The listing builds one solid part. Answer for the finished solid, in the listing's coordinates (mm). Face numbers are marked on the shaded views. A direction names the side the tool comes from. Round coordinates to 2 decimals unless told otherwise and drop trailing zeros. Write each loop counter-clockwise with the first axis right and the second up, starting at its lowest first coordinate (ties: lowest second). Pieces come first, ordered by that corner, then holes.
(1) Each of these flat-tipped pins is pushed along its axis until it touches: pin 1 Ø1 at (x, z) = (-41.5, -9.5) entering from +Y; pin 2 Ø8 at (y, z) = (-8.5, 13) entering from +X. Where does it stop, or does it pass through?
(2) For the marked faces 1 and 2, determine the directions among +Z, -Z, +X, -X, +Y, -Y from which every point of the face is accessible in a straight line to the end or side of a thin tool.
(3) A cutting plane is placed at D-D, the plane x = -24. Give the vertices of the cut face in (y, z).
(4) Find the intervals of material crossed by probe 1 along Z at (x, y) = (30.5, -5.25); probe 2 along Y at (x, z) = (38, 11); probe 3 along Y at (x, z) = (0, -23), in increasing order.
(5) A cutting plane is placed at A-A, the plane z = -8.5. Give the vertices of the cut face in (x, y), and give its area (3 significant figures).
(6) A cutting plane is placed at B-B, the plane y = -5.5. Give the vertices of the cut face in (x, z), and give its area (3 significant figures).
(7) The mould has two halves that part along Y. Classify the marked faces 3, 4 and 5: +Y half, -Y half, draft (parallel to the pull), parting line (faces both ways), or undercut.
(8) A cutting plane is placed at C-C, the plane x = 38.5. Give the vertices of the cut face in (y, z).
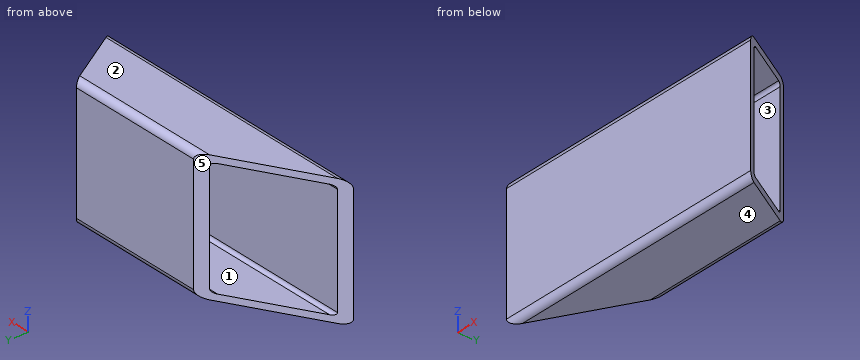
from build123d import *

# Parameters (mm, degrees)
F0_W     = 112.7125
F0_H     = 50.8
F1_DEPTH = 12.7
F2_T     = -2.54
F4_DEPTH = 50.801
F6_DEPTH = 50.801
F7_R     = 2.54
F8_R     = 1.27


with BuildPart() as f1:
    # F0 (on Front) → F1 (new body, symmetric)
    with BuildSketch(Plane.XZ):
        Rectangle(F0_W, F0_H)
    extrude(amount=F1_DEPTH, both=True)

    # F2
    f2_openings = [f1.faces().sort_by_distance(p)[0] for p in [
        (-56.35625, 0, 0),
        (56.35625, 0, 0),
    ]]
    offset(amount=F2_T, openings=f2_openings)

    # F3 (on face) → F4 (cut, through all)
    with BuildSketch(Plane(origin=(0, 0, -25.4), x_dir=(1, 0, 0), z_dir=(0, 0, -1))):
        Polygon((-12.3621594878, -12.7), (-56.35625, 12.7), (-56.35625, -12.7), align=None)
    extrude(amount=-F4_DEPTH, mode=Mode.SUBTRACT)

    # F5 (on face) → F6 (cut, through all)
    with BuildSketch(Plane.XY.offset(25.4)):
        Polygon((41.6915531626, 12.7), (56.35625, -12.7), (56.35625, 12.7), align=None)
    extrude(amount=-F6_DEPTH, mode=Mode.SUBTRACT)

    # F7
    f7_edges = [f1.edges().sort_by_distance(p)[0] for p in [
        (0, -12.7, 25.4),
        (14.664697, 12.7, 25.4),
        (14.664697, 12.7, -25.4),
        (0, -12.7, -25.4),
    ]]
    fillet(f7_edges, radius=F7_R)

    # F8
    f8_edges = [f1.edges().sort_by_distance(p)[0] for p in [
        (13.198227, 10.16, 22.86),
        (1.46647, -10.16, 22.86),
        (1.46647, -10.16, -22.86),
        (13.198227, 10.16, -22.86),
    ]]
    fillet(f8_edges, radius=F8_R)


solid = f1.part
Solutions:
1. pin 1: stops at y = -10.16
1. pin 2: stops at x = 56.24
2. face 1: +X, -X
2. face 2: +Z, +X, -X, +Y, -Y
3. outline: (-12.7, -22.86) arc R2.54 ccw to (-10.16, -25.4) - (5.98, -25.4) - (5.98, -22.86) - (-8.89, -22.86) arc R1.27 cw to (-10.16, -21.59) - (-10.16, 21.59) arc R1.27 cw to (-8.89, 22.86) - (5.98, 22.86) - (5.98, 25.4) - (-10.16, 25.4) arc R2.54 ccw to (-12.7, 22.86) - close
4. probe 1: z = -25.4 to -22.86, 22.86 to 25.4
4. probe 2: y = -12.7 to -10.16, 10.16 to 12.7
4. probe 3: y = -12.7 to 12.7
5. outline: (-56.36, -12.7) - (56.36, -12.7) - (54.89, -10.16) - (-51.96, -10.16) - close; (-16.76, 10.16) - (43.16, 10.16) - (41.69, 12.7) - (-12.36, 12.7) - close
5. area: 424 mm2
6. outline: (-43.89, -25.4) - (52.2, -25.4) - (52.2, -22.86) - (-43.89, -22.86) - close; (-43.89, 22.86) - (52.2, 22.86) - (52.2, 25.4) - (-43.89, 25.4) - close
6. area: 488 mm2
7. face 3: undercut
7. face 4: draft
7. face 5: +Y half
8. outline: (-12.7, -22.86) arc R2.54 ccw to (-10.16, -25.4) - (10.16, -25.4) arc R2.54 ccw to (12.7, -22.86) - (12.7, 22.86) arc R2.54 ccw to (10.16, 25.4) - (-10.16, 25.4) arc R2.54 ccw to (-12.7, 22.86) - close; hole (-10.16, -21.59) arc R1.27 ccw to (-8.89, -22.86) - (8.89, -22.86) arc R1.27 ccw to (10.16, -21.59) - (10.16, 21.59) arc R1.27 ccw to (8.89, 22.86) - (-8.89, 22.86) arc R1.27 ccw to (-10.16, 21.59) - close
